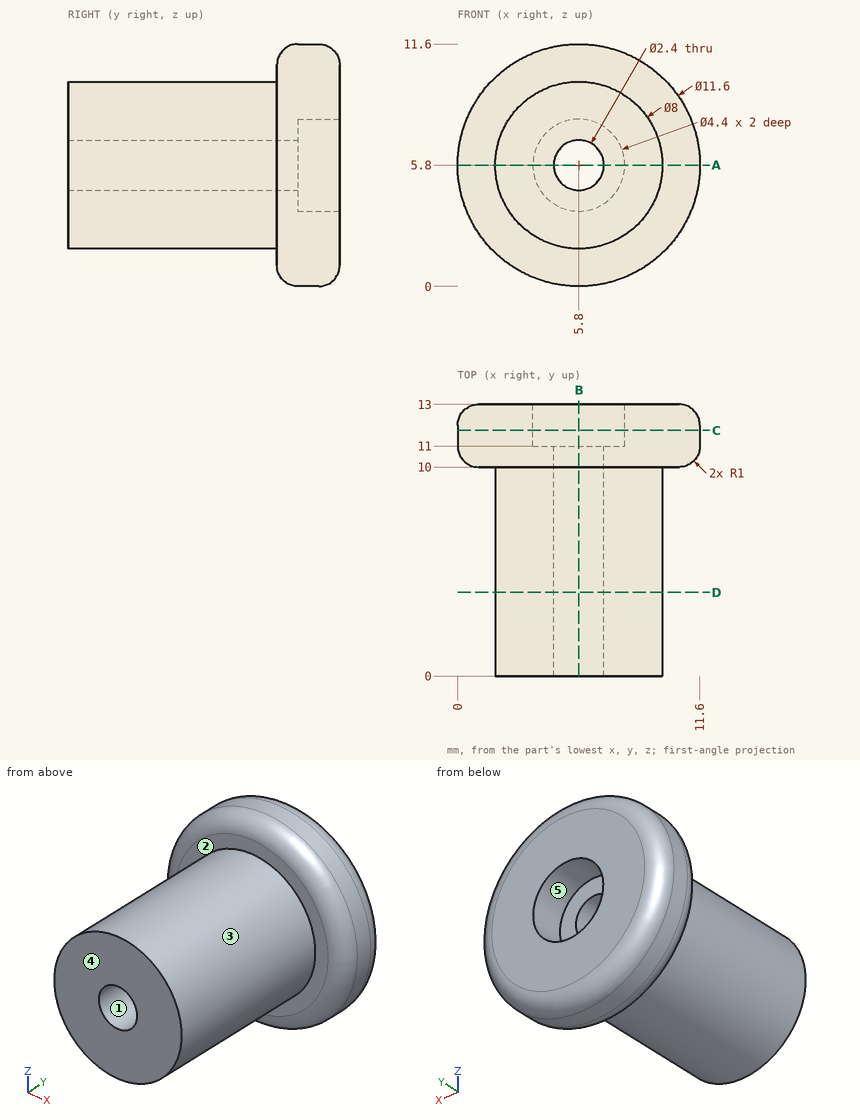
Verification items for this drawing (mm, ordinates from the low corner). A direction names the side the tool comes from. Give positions to 0.01 mm unless a question says otherwise; leave off trailing zeros. Write each loop counter-clockwise with the first axis right and the second up, starting at its lowest first coordinate (ties: lowest second). Pieces come first, ordered by that corner, then holes. Notation, with made-up numbers: (83.25, 58) - (104.25, 58) arc R24 ccw to (104.25, 87) - close; hole circle Ø4 at (-25, -8.75). An arc over 180 degrees is marked (long way). Answer as CSV lines item,"result". Start each with the question number.
1. Draft check along X on the marked faces 3, 4 and 5. Enter one of: pulls with the +X half, pulls with the -X half, needs draft (parallel to the pull), parting line crosses it, or undercut.
2. Sectioned sample at B-B (x = 5.8). Record the boundary of the cut face in (y, z).
3. Sectioned sample at C-C (y = 11.75). Record the boundary of the cut face in (x, z), then the cut area to 3 significant figures.
4. Set-up check for the marked faces 1 and 2: record each of +Z, -Z, +X, -X, +Y, -Y from which the full face is reachable in a straight line by a thin tool's end or side.
5. Sectioned sample at A-A (z = 5.8). Record the boundary of the cut face in (x, y), then the cut area to 3 significant figures.
6. Depth check by flat-ended pin: pin 1 (4 mm diameter, centred on x = 5.8, z = 5.8, fed in from +Y); pin 2 (5 mm diameter, centred on x = 8, y = 4.5, fed in from +Z); pin 3 (2 mm diameter, centred on x = 10, z = 1, fed in from -Y); pin 4 (3 mm diameter, centred on x = 7, z = 3.5, fed in from -Y). Enter the tip coordinate at first touch or a pass-through.
7. Sectioned sample at D-D (y = 4). Record the boundary of the cut face in (x, z), then the cut area to 3 significant figures.
8. Thickness scan on line 1 (X direction, y = 5.25, z = 5.8); line 2 (X direction, y = 11.5, z = 6.5); line 3 (Y direction, x = 4, z = 1.25). Record the ranges inside material, lowest first.
Derived:
1,face 3,"parting line crosses it"
1,face 4,"needs draft"
1,face 5,"undercut"
2,outline,"(0, 1.8) - (10, 1.8) - (10, 1) arc R1 ccw to (11, 0) - (12, 0) arc R1 ccw to (13, 1) - (13, 3.6) - (11, 3.6) - (11, 4.6) - (0, 4.6) - close; (0, 7) - (11, 7) - (11, 8) - (13, 8) - (13, 10.6) arc R1 ccw to (12, 11.6) - (11, 11.6) arc R1 ccw to (10, 10.6) - (10, 9.8) - (0, 9.8) - close"
3,outline,"circle Ø11.6 at (5.8, 5.8); hole circle Ø4.4 at (5.8, 5.8)"
3,area,"90.5 mm²"
4,face 1,"+Y, -Y"
4,face 2,"-Y"
5,outline,"(0, 11) arc R1 ccw to (1, 10) - (1.8, 10) - (1.8, 0) - (4.6, 0) - (4.6, 11) - (3.6, 11) - (3.6, 13) - (1, 13) arc R1 ccw to (0, 12) - close; (7, 0) - (9.8, 0) - (9.8, 10) - (10.6, 10) arc R1 ccw to (11.6, 11) - (11.6, 12) arc R1 ccw to (10.6, 13) - (8, 13) - (8, 11) - (7, 11) - close"
5,area,"78.7 mm²"
6,pin 1,"y = 11"
6,pin 2,"z = 9.8"
6,pin 3,"y = 10.18"
6,pin 4,"y = 0"
7,outline,"circle Ø8 at (5.8, 5.8); hole circle Ø2.4 at (5.8, 5.8)"
7,area,"45.7 mm²"
8,line 1,"1.8 to 4.6, 7 to 9.8"
8,line 2,"0.04 to 3.71, 7.89 to 11.56"
8,line 3,"10 to 13"
